The model under review builds one solid part; all positions refer to its coordinate system, in mm. Face numbers are marked on the shaded views. A direction names the side the tool comes from. Round coordinates to 2 decimals unless told otherwise and drop trailing zeros. Write each loop counter-clockwise with the first axis right and the second up, starting at its lowest first coordinate (ties: lowest second). Pieces come first, ordered by that corner, then holes.
Item 1: Add section B-B (x = 77). Give the boundary of the cut face in (y, z).
Item 2: Add section D-D (z = -42). Give the boundary of the cut face in (x, y).
Item 3: Clearance check with flat-ended pins moving along their axes: pin 1 Ø1.5 at (x, y) = (-14.5, -10.5) entering from +Z; pin 2 Ø6 at (x, y) = (45, 0.5) entering from -Z; pin 3 Ø3 at (y, z) = (14, 0) entering from +X. State where each tip first meets the part, or that it passes through.
Item 4: Machinability: for the marked faces 1, 2, 3, 4 and 5, which of the approach directions +Z, -Z, +X, -X, +Y, -Y give a long, thin tool a straight path to every point of the face, cutting with its end or side? Answer none if there is none.
Item 5: To check wall thickness, follow L1, parallel to Z at x = -46, y = 16; L2, parallel to Y at x = -90, z = -16.5; L3, parallel to Z at x = 132.5, y = 18.5. State the ranges of each line that lie inside material, in increasing order.
Item 6: Add section C-C (y = 20.5). Give the boundary of the cut face in (x, z), plus the area to 3 significant figures.
Item 7: Add section A-A (y = -6). Give the boundary of the cut face in (x, z), plus the area to 3 significant figures.
```python
from build123d import *

# Parameters (mm, degrees)
BOSS_EXTRUDE1_DEPTH = 60
SKETCH2_R           = 15
BOSS_EXTRUDE2_DEPTH = 70
BOSS_EXTRUDE3_START = 70
SKETCH3_R           = 15
BOSS_EXTRUDE3_DEPTH = 70
SKETCH4_W           = 60
SKETCH4_H           = 40
CUT_EXTRUDE1_DEPTH  = 75
SKETCH5_R           = 15
CUT_EXTRUDE2_DEPTH  = 75


with BuildPart() as part:
    # Sketch1 → Boss-Extrude1 (new body)
    with BuildSketch(Plane.XY):
        with BuildLine():
            Line((-91.343193625, 24.62689066), (128.656806375, 24.62689066))
            ThreePointArc((128.656806375, 24.62689066), (153.656806375, -0.37310934), (128.656806375, -25.37310934))
            Line((128.656806375, -25.37310934), (-91.343193625, -25.37310934))
            ThreePointArc((-91.343193625, -25.37310934), (-116.343193625, -0.37310934), (-91.343193625, 24.62689066))
        make_face()
    extrude(amount=BOSS_EXTRUDE1_DEPTH)

    # Sketch2 → Boss-Extrude2 (add)
    with BuildSketch(Plane.XY.offset(60)):
        with Locations((-91.343193625, -0.37310934)):
            Circle(SKETCH2_R)
    extrude(amount=BOSS_EXTRUDE2_DEPTH)

    # Sketch3 → Boss-Extrude3 (add)
    with BuildSketch(Plane(origin=(0, 0, 0), x_dir=(-1, 0, 0), z_dir=(0, 0, -1)).offset(BOSS_EXTRUDE3_START)):
        with Locations(Location((91.343193625, -0.37310934, 0), (0, 0, 180))):
            Circle(SKETCH3_R)
    extrude(amount=-BOSS_EXTRUDE3_DEPTH)

    # Sketch4 → Cut-Extrude1 (cut)
    with BuildSketch(Plane(origin=(0, 24.62689066, 0), x_dir=(1, 0, 0), z_dir=(0, 1, 0))):
        with Locations((123.656806375, -30)):
            Rectangle(SKETCH4_W, SKETCH4_H)
    extrude(amount=-CUT_EXTRUDE1_DEPTH, mode=Mode.SUBTRACT)

    # Sketch5 → Cut-Extrude2 (cut)
    with BuildSketch(Plane.XY.offset(60)):
        with Locations((128.656806375, -0.37310934)):
            Circle(SKETCH5_R)
    extrude(amount=-CUT_EXTRUDE2_DEPTH, mode=Mode.SUBTRACT)


solid = part.part
```
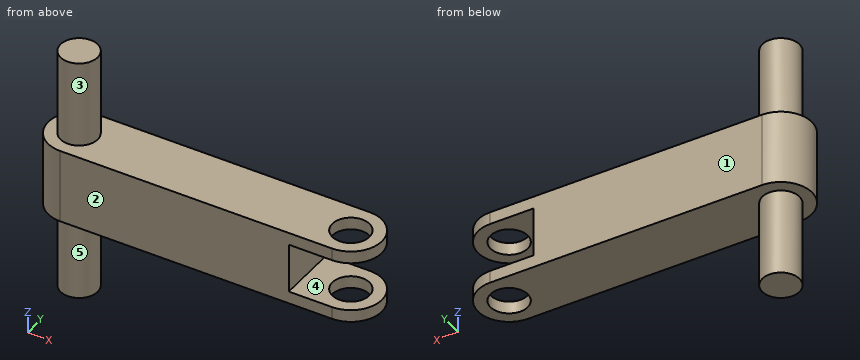
Numbers:
1. outline: (-25.37, 0) - (24.63, 0) - (24.63, 60) - (-25.37, 60) - close
2. outline: circle Ø30 at (-91.34, -0.37)
3. pin 1: stops at z = 60
3. pin 2: stops at z = 0
3. pin 3: stops at x = 150.09
4. face 1: +Z, -Z, +X, -X, +Y
4. face 2: +Z, -Z, +X, -X, -Y
4. face 3: +Z
4. face 4: +X, +Y, -Y
4. face 5: -Z
5. L1: z = 0 to 60
5. L2: y = -15.31 to 14.57
5. L3: z = 0 to 10, 50 to 60
6. outline: (-105.1, 0) - (142.42, 0) - (142.42, 10) - (93.66, 10) - (93.66, 50) - (142.42, 50) - (142.42, 60) - (-105.1, 60) - close
6. area: 12,900 mm2
7. outline: (-115.7, 0) - (-105.25, 0) - (-105.25, -70) - (-77.44, -70) - (-77.44, 0) - (114.75, 0) - (114.75, 10) - (93.66, 10) - (93.66, 50) - (114.75, 50) - (114.75, 60) - (-77.44, 60) - (-77.44, 130) - (-105.25, 130) - (-105.25, 60) - (-115.7, 60) - close; (142.56, 0) - (153.02, 0) - (153.02, 10) - (142.56, 10) - close; (142.56, 50) - (153.02, 50) - (153.02, 60) - (142.56, 60) - close
7. area: 17,100 mm2
